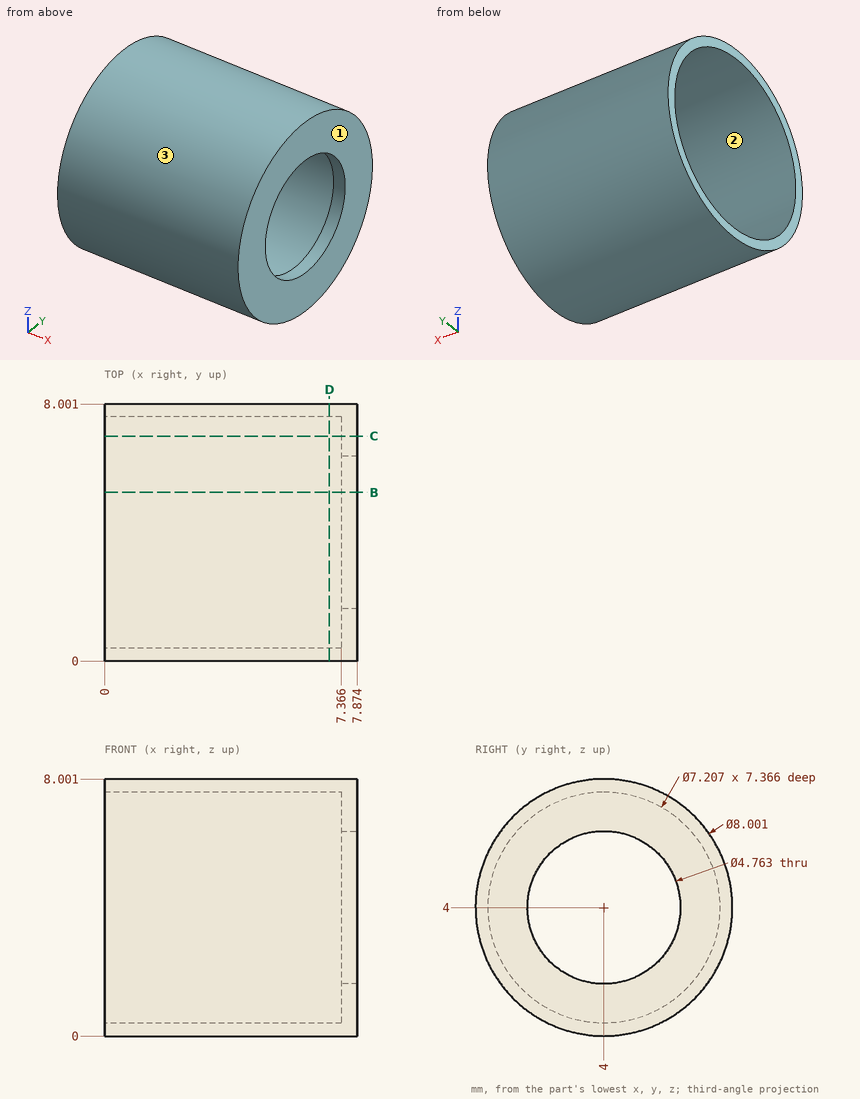
The drawing under review shows one solid part. Ordinate dimensions are in mm from its lowest x, y, z. Give positions to 0.01 mm unless a question says otherwise; leave off trailing zeros. Loops run counter-clockwise (first coordinate to the right, second up) from the corner with the lowest first, then second, coordinate; pieces in that order, holes last. Notation, with made-up numbers: M 22.5,42 L 67.5,42 A7 cw 67.5,55 Z; hole C 37.25,66 d10. An arc over 180 degrees is marked long. Return JSON: item names as keys, results as strings. Group by question number.
Item 1: Insertion check: pin 1 Ø2 at (y, z) = (4, 2) entering from -X; pin 2 Ø3 at (x, y) = (4.5, 7) entering from -Z. Each pin has a flat end and moves straight along its axis. Give the tip position at first contact, or say it passes through.
Item 2: We need section C-C (y = 7). Give the boundary of the cut face in (x, z) (1 decimal).
Item 3: For probe 1 along X at (y, z) = (4.75, 1.25) (1 decimal); probe 2 along Y at (x, z) = (5.5, 4) (1 decimal), list the stretches that pass through material, from the lowest coordinate up.
Item 4: Mouldability with a two-part tool opening along Y and no side actions: class the marked faces 1, 2 and 3 as released by +Y, released by -Y, zero draft, split by the parting line, or undercut.
Item 5: We need section D-D (x = 7). Give the boundary of the cut face in (y, z) (1 decimal).
Item 6: We need section B-B (y = 5.25). Give the boundary of the cut face in (x, z) (1 decimal).
Output:
{
 "1": {"pin 1": "stops at x = 7.37", "pin 2": "stops at z = 0.29"},
 "2": {"outline": "M 0,1.4 L 7.9,1.4 L 7.9,6.6 L 0,6.6 L 0,6 L 7.4,6 L 7.4,2 L 0,2 Z"},
 "3": {"probe 1": "x = 7.4 to 7.9", "probe 2": "y = 0 to 0.4, 7.6 to 8"},
 "4": {"face 1": "zero draft", "face 2": "undercut", "face 3": "split by the parting line"},
 "5": {"outline": "C 4,4 d8; hole C 4,4 d7.2"},
 "6": {"outline": "M 0,0.2 L 7.9,0.2 L 7.9,2 L 7.4,2 L 7.4,0.6 L 0,0.6 Z; M 0,7.4 L 7.4,7.4 L 7.4,6 L 7.9,6 L 7.9,7.8 L 0,7.8 Z"}
}
